Here's how the part is built. I have some questions about the finished solid (model axes, mm). Coordinates: 2 decimals unless noted, no trailing zeros. Write each loop counter-clockwise with the first axis right and the second up, starting at its lowest first coordinate (ties: lowest second). Pieces come first, ordered by that corner, then holes.
Item 1: I'm going to push flat-ended pins straight in: P1, Ø6, axis at x = 8, y = -535, coming from the -Z side; P2, Ø12, axis at y = -169, z = 18.5, coming from the -X side; P3, Ø1.5, axis at x = -14.5, z = -7, coming from the -Y side. Where does each tip first touch, or does it pass through?
Item 2: I want a section at C-C (y = -193.5). Please give me the cut outline in (x, z).
Item 3: Please list where these lines run through material, in increasing order: line 1 (Y direction, x = -15.5, z = -14); line 2 (Y direction, x = 7.5, z = -11); line 3 (X direction, y = -415.5, z = -0.5).
Item 4: I want a section at B-B (x = 0). Please give me the cut outline in (y, z), and give its area (3 significant figures).
Item 5: I want a section at A-A (z = 0). Please give me the cut outline in (x, y).
from build123d import *

# Parameters (mm, degrees)
F0_R     = 19.05
F1_DEPTH = 584.2
F3_R     = 25.4
F4_DEPTH = 6.35
F2_R     = 25.4
F2_R_2   = 19.05
F5_DEPTH = 6.35
F6_R     = 12.7
F7_DEPTH = 25.4
F8_R     = 12.7
F9_DEPTH = 25.4


with BuildPart() as f1:
    # F0 (on Front) → F1 (new body)
    with BuildSketch(Plane.XZ):
        Circle(F0_R)
    extrude(amount=F1_DEPTH)

    # F3 (on face) → F4 (join)
    with BuildSketch(Plane.XZ.offset(584.2)):
        Circle(F3_R)
    extrude(amount=-F4_DEPTH)

    # F2 (on face) → F5 (join)
    with BuildSketch(Plane(origin=(0, 0, 0), x_dir=(-1, 0, 0), z_dir=(0, 1, 0))):
        Circle(F2_R)
        Circle(F2_R_2, mode=Mode.SUBTRACT)
    extrude(amount=-F5_DEPTH)

    # F6 (on face) → F7 (join)
    with BuildSketch(Plane.XZ.offset(584.2)):
        Circle(F6_R)
    extrude(amount=F7_DEPTH)

    # F8 (on face) → F9 (join)
    with BuildSketch(Plane(origin=(0, 0, 0), x_dir=(-1, 0, 0), z_dir=(0, 1, 0))):
        Circle(F8_R)
    extrude(amount=F9_DEPTH)


solid = f1.part
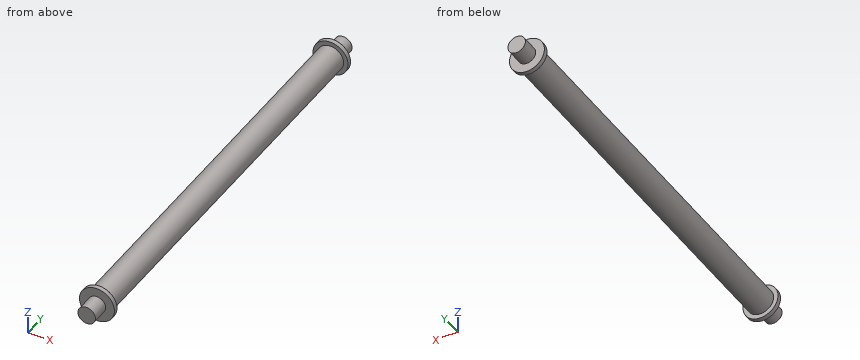
Answer:
1. P1: stops at z = -18.38
1. P2: stops at x = -14.38
1. P3: stops at y = -584.2
2. outline: circle Ø38.1 at (0, 0)
3. line 1: y = -584.2 to -577.85, -6.35 to 0
3. line 2: y = -584.2 to 0
3. line 3: x = -19.04 to 19.04
4. outline: (-609.6, -12.7) - (-584.2, -12.7) - (-584.2, -25.4) - (-577.85, -25.4) - (-577.85, -19.05) - (-6.35, -19.05) - (-6.35, -25.4) - (0, -25.4) - (0, -12.7) - (25.4, -12.7) - (25.4, 12.7) - (0, 12.7) - (0, 25.4) - (-6.35, 25.4) - (-6.35, 19.05) - (-577.85, 19.05) - (-577.85, 25.4) - (-584.2, 25.4) - (-584.2, 12.7) - (-609.6, 12.7) - close
4. area: 23,700 mm2
5. outline: (-25.4, -584.2) - (-12.7, -584.2) - (-12.7, -609.6) - (12.7, -609.6) - (12.7, -584.2) - (25.4, -584.2) - (25.4, -577.85) - (19.05, -577.85) - (19.05, -6.35) - (25.4, -6.35) - (25.4, 0) - (12.7, 0) - (12.7, 25.4) - (-12.7, 25.4) - (-12.7, 0) - (-25.4, 0) - (-25.4, -6.35) - (-19.05, -6.35) - (-19.05, -577.85) - (-25.4, -577.85) - close
